Could you check a few things on this model? Use its own coordinates, in mm. A direction names the side the tool comes from. Give positions to 0.01 mm unless a question says otherwise; leave off trailing zeros. Use a Markdown table: item, result. Add a question column.
Item 1: Suppose I cut it at A-A on y = -21. Count the separate pieces of the cut face and the enclosed holes in it, plus the area to 3 significant figures.
Item 2: For faces 4 (the face through (-3.54, -19.72, 44.274)), 5 (the face through (11.612, -22, 25)), 6 (the face through (-26, -40, 5)), which set-ups out of +Z, -Z, +X, -X, +Y, -Y let a thin tool reach every point of the face, with its end or its side?
Item 3: If I drill on L1, parallel to X at y = -12.5, z = 20; L2, parallel to Z at x = -15.5, y = -13; L3, parallel to X at y = -7, z = 35, over which ranges is the centre line in solid material (lowest first)? Write a range as from..to.
Item 4: If we mould it in two halves opening along Z, with no side actions, what happens to faces 1 (the face through (-127.94, -0.9, 17.65)), 2 (the face through (6, 0, -5)), 3 (the face through (112.27, -21.75, 57.21))? For each: released by +Z, released by -Z, zero draft, split by the parting line, or undercut.
Item 5: I'm going to push flat-ended pins straight in: pin 1 Ø10 at (x, z) = (37.5, -116) entering from -Y; pin 2 Ø8 at (x, y) = (-39, -29) entering from -Z; pin 3 Ø20.5 at (y, z) = (-12.5, 24.5) entering from +X. Where does each tip first touch, or does it pass through?
from build123d import *

# Parameters (mm, degrees)
F1_DEPTH = 40
F2_T     = -4
F3_R     = 3
F4_R     = 5
F5_DEPTH = 50


with BuildPart() as f1:
    # F0 (on Front) → F1 (new body)
    with BuildSketch(Plane.XZ):
        Polygon((26.7151626776, -158.4525242576), (158.9527449935, -23.5568932488), (71.5230363335, 143.8935635605), (-114.7490775608, 112.4880062915), (-142.4418664438, -74.3721523457), align=None)
        Polygon((-14.3848736808, 50.5347126111), (7.6121715753, 37.8347126111), (7.6121715753, 12.4347126111), (-14.3848736808, -0.2652873889), (-36.381918937, 12.4347126111), (-36.381918937, 37.8347126111), align=None, mode=Mode.SUBTRACT)
    extrude(amount=F1_DEPTH)

    # F2
    f2_openings = [f1.faces().sort_by_distance(p)[0] for p in [
        (0.403766, -40, -0.705501),
    ]]
    offset(amount=F2_T, openings=f2_openings, kind=Kind.INTERSECTION)

    # F3
    f3_edges = [f1.edges().sort_by_distance(p)[0] for p in [
        (-57.863352, 0, -116.412338),
        (92.833954, 0, -91.004709),
        (-128.595472, 0, 19.057927),
        (-21.613021, 0, 128.190785),
        (115.237891, 0, 60.168335),
        (71.523036, -20, 143.893564),
        (-114.749078, -20, 112.488006),
        (-142.441866, -20, -74.372152),
        (26.715163, -20, -158.452524),
        (158.952745, -20, -23.556893),
        (69.322328, -22, 139.466069),
        (-111.218337, -22, 109.026837),
        (-138.05904, -22, -72.083778),
        (154.061891, -22, -22.832066),
        (25.893158, -22, -153.577062),
    ]]
    fillet(f3_edges, radius=F3_R)

    # F4 (on face) → F5 (join)
    with BuildSketch(Plane.XZ.offset(4)):
        with Locations((0, -68.4551969171)):
            Circle(F4_R)
    extrude(amount=F5_DEPTH)


solid = f1.part
Findings below:
| question | item | result |
|---|---|---|
| 1 | separate pieces | 3 |
| 1 | enclosed holes | 2 |
| 1 | area | 4,460 mm^2 |
| 2 | face 4 | +Y, -Y |
| 2 | face 5 | -Y |
| 2 | face 6 | +Z, +X, -X, -Y |
| 3 | L1 | x = -128.46..-124.41, -40.38..-36.38, 7.61..11.61, 131.7..136.21 |
| 3 | L2 | z = -137.47..-133, -4.24..0.38, 49.89..54.51, 125.16..129.22 |
| 3 | L3 | x = -126.23..-122.19, -40.38..-36.38, 7.61..11.61, 123.87..128.38 |
| 4 | face 1 | released by +Z |
| 4 | face 2 | zero draft |
| 4 | face 3 | undercut |
| 5 | pin 1 | stops at y = -4 |
| 5 | pin 2 | stops at z = -127.78 |
| 5 | pin 3 | stops at x = 139.21 |
